Input: part model. Units: mm. Frame: model coordinates. Coordinates: 2 decimals unless noted, no trailing zeros. Loops run counter-clockwise (first coordinate to the right, second up) from the corner with the lowest first, then second, coordinate; pieces in that order, holes last. Notation, with made-up numbers: (-8, -36) - (34, -36) arc R14 cw to (34, -11) - close; hole circle Ø6 at (-14.5, 8). An arc over 180 degrees is marked (long way). Use one line per item in the form item = value.
from build123d import *


# Read off the part's stored shape, not the designer's step: Thicken2
with BuildPart() as part:
    # Thicken2 outline → Thicken2 (revolve)
    with BuildSketch(Plane(origin=(-5.431630681, 0, 0), x_dir=(1, 0, 0), z_dir=(0, 0, 1))):
        Polygon((4.120349674, 1.929400611), (4.136521177, -0.904564978), (4.936508153, -0.9), (4.918558927, 2.245501685), (3.3, 3.988409531), (3.3, 4.088409531), (5, 5.913409531), (3.3, 7.738409531), (3.3, 7.838409531), (5, 9.663409531), (3.3, 11.488409531), (3.3, 11.588409531), (5, 13.413409531), (3.3, 15.238409531), (3.3, 15.338409531), (5, 17.163409531), (3.3, 18.988409531), (3.3, 19.088409531), (5, 20.913409531), (3.3, 22.738409531), (3.3, 22.838409531), (5, 24.663409531), (3.3, 26.488409531), (3.3, 26.588409531), (5, 28.413409531), (3.3, 30.238409531), (3.3, 30.338409531), (5, 32.163409531), (3.3, 33.988409531), (3.3, 34.102954004), (0, 34.102954004), (0, 33.302954004), (2.845194483, 33.302954004), (3.906687965, 32.163409531), (2.5, 30.653288628), (2.5, 29.923530434), (3.906687965, 28.413409531), (2.5, 26.903288628), (2.5, 26.173530434), (3.906687965, 24.663409531), (2.5, 23.153288628), (2.5, 22.423530434), (3.906687965, 20.913409531), (2.5, 19.403288628), (2.5, 18.673530434), (3.906687965, 17.163409531), (2.5, 15.653288628), (2.5, 14.923530434), (3.906687965, 13.413409531), (2.5, 11.903288628), (2.5, 11.173530434), (3.906687965, 9.663409531), (2.5, 8.153288628), (2.5, 7.423530434), (3.906687965, 5.913409531), (2.5, 4.403288628), (2.5, 3.674236782), align=None)
    revolve(axis=Axis((-5.431630681, 0, 0), (0, 1, 0)))


solid = part.part
Q1. First-contact query: P1, Ø3, axis at y = 19, z = 3.5, coming from the +X side; P2, Ø6, axis at x = -5.43, z = 0, coming from the -Y side; P3, Ø4.5, axis at x = -5.43, z = 0, coming from the -Y side. Flat tips, straight axial feed; report the tip coordinate or a pass-through.
Check values:
P1 = -1.87
P2 = 3.13
P3 = 33.3
Q2. Ray query, line 1 along Y through (x, z) = (-6.75, 0.25); line 2 along X through (y, z) = (26, -0.75); line 3 along X through (y, z) = (14, -2.5). Return the intervals inside material, ascending. Write a range as [from, to].
Check values:
line_1 = [33.3, 34.1]
line_2 = [-9.11, -7.99], [-2.88, -1.75]
line_3 = [-9.12, -7.68], [-3.19, -1.75]
Q3. Cut plane A-A, the plane y = 31.5. Return loops of the section in (x, z), then the cut area to 3 significant figures.
Check values:
outline = circle Ø8.76 at (-5.43, 0); hole circle Ø6.58 at (-5.43, 0)
area = 26.3 mm²
